The model under review builds one solid part; all positions refer to its coordinate system, in mm. Face numbers are marked on the shaded views. A direction names the side the tool comes from. Coordinates: 2 decimals unless noted, no trailing zeros. Order: outer loops, then holes, each group sorted by start corner. A loop starts at its lowest first (then second) coordinate and runs counter-clockwise, first axis right, second up. Notation, with made-up numbers: (46, 9.5) - (57, 9.5) arc R29 ccw to (57, 42.5) - close; hole circle Ø1 at (-9.75, 41). An arc over 180 degrees is marked (long way). Answer in a Markdown table with one row per item.
```python
from build123d import *

# Parameters (mm, degrees)
BOSS_EXTRUDE1_DEPTH          = 44.45
FILLET2_R                    = 6.35
CUT_EXTRUDE1_START           = -22.225
CUT_EXTRUDE1_DEPTH           = 22.225
FILLET3_R                    = 2.54
F_3_8_0_375_DIAMETER_HOLE1_D = 10.16


with BuildPart() as part:
    # Sketch1 → Boss-Extrude1 (new body)
    with BuildSketch(Plane.XY):
        with BuildLine():
            Line((0, 0), (57.15, 0))
            Line((57.15, 0), (57.15, -9.525))
            Line((57.15, -9.525), (0, -11.7445024))
            Line((0, -11.7445024), (-20.4502, -11.7445024))
            Line((-20.4502, -11.7445024), (-20.4502, 9.8454976))
            Line((-20.4502, 9.8454976), (-48.3902, 9.8454976))
            Line((-48.3902, 9.8454976), (-48.3902, 20.0054976))
            ThreePointArc((-48.3902, 20.0054976), (-44.670456121, 28.985753721), (-35.6902, 32.7054976))
            Line((-35.6902, 32.7054976), (-22.9902, 32.7054976))
            Line((-22.9902, 32.7054976), (-6.35, 57.15))
            Line((-6.35, 57.15), (0, 57.15))
            Line((0, 57.15), (0, 0))
        make_face()
    extrude(amount=BOSS_EXTRUDE1_DEPTH)

    # Fillet2
    fillet2_edges = [part.edges().sort_by_distance(p)[0] for p in [
        (0, 0, 22.225),
    ]]
    fillet(fillet2_edges, radius=FILLET2_R)

    # Sketch3 → Cut-Extrude1 (cut)
    with BuildSketch(Plane.XY.offset(44.45).offset(CUT_EXTRUDE1_START)):
        with BuildLine():
            Line((-48.3902, 9.8454976), (-20.4502, 9.8454976))
            Line((-20.4502, 9.8454976), (-20.4502, 36.436765018))
            Line((-20.4502, 36.436765018), (-22.9902, 32.7054976))
            Line((-22.9902, 32.7054976), (-35.6902, 32.7054976))
            ThreePointArc((-35.6902, 32.7054976), (-44.670456121, 28.985753721), (-48.3902, 20.0054976))
            Line((-48.3902, 20.0054976), (-48.3902, 9.8454976))
        make_face()
    extrude(amount=CUT_EXTRUDE1_DEPTH, mode=Mode.SUBTRACT)

    # Fillet3
    fillet3_edges = [part.edges().sort_by_distance(p)[0] for p in [
        (-22.9902, 32.7054976, 11.1125),
    ]]
    fillet(fillet3_edges, radius=FILLET3_R)

    # 3/8 (0.375) Diameter Hole1 (through all)
    with Locations(Plane(origin=(0, 0, 0), x_dir=(-1, 0, 0), z_dir=(0, 0, -1))):
        with Locations((35.6902, 21.2754976)):
            Hole(F_3_8_0_375_DIAMETER_HOLE1_D / 2)


solid = part.part
```
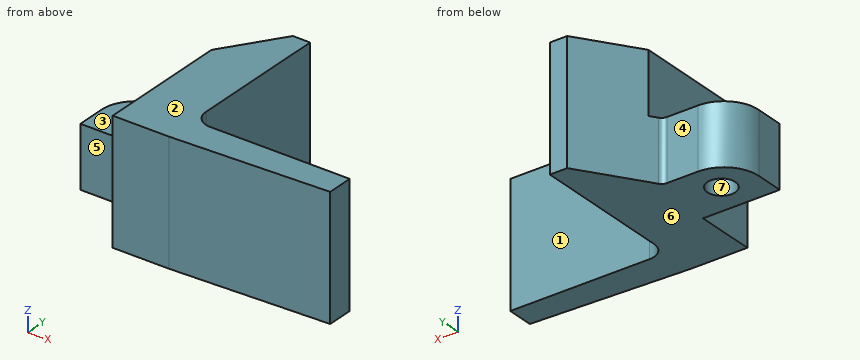
Item 1: Mouldability with a two-part tool opening along Y and no side actions: class the marked faces 4, 5, 6 and 7 as +Y half, -Y half, draft (parallel to the pull), parting line (faces both ways), or undercut.
Check values:
| item | result |
|---|---|
| face 4 | +Y half |
| face 5 | -Y half |
| face 6 | draft |
| face 7 | undercut |
Item 2: We need section A-A, the plane x = -38. Write out the cut boundary in (y, z) (1 decimal).
Check values:
| item | result |
|---|---|
| outline | (9.8, 0) - (16.8, 0) - (16.8, 22.2) - (9.8, 22.2) - close; (25.8, 0) - (32.5, 0) - (32.5, 22.2) - (25.8, 22.2) - close |
Item 3: Clearance check with flat-ended pins moving along their axes: pin 1 Ø12.5 at (x, z) = (-27.5, 16.5) entering from +Y; pin 2 Ø1 at (x, y) = (-17, 39.5) entering from -Z; pin 3 Ø4 at (y, z) = (35, 7.5) entering from -X; pin 4 Ø2 at (x, z) = (35.5, 31.5) entering from -Y. State where each tip first meets the part, or that it passes through.
Check values:
| item | result |
|---|---|
| pin 1 | y = 35.26 |
| pin 2 | z = 0 |
| pin 3 | x = -23.15 |
| pin 4 | y = -10.4 |
Item 4: To check wall thickness, follow line 1 (X direction, y = -6.5, z = 16); line 2 (X direction, y = 23, z = 38.5); line 3 (Y direction, x = 14, z = 11.5). State the ranges of each line that lie inside material, in increasing order. Write a range as from..to.
Check values:
| item | result |
|---|---|
| line 1 | -20.45..57.15 |
| line 2 | -20.45..0 |
| line 3 | -11.2..0 |
Item 5: We need section C-C, the plane y = -1.5. Write out the cut boundary in (x, z).
Check values:
| item | result |
|---|---|
| outline | (-20.45, 0) - (57.15, 0) - (57.15, 44.45) - (-20.45, 44.45) - close |
Item 6: Tool access review of the marked faces 1, 2 and 3: name each direction out of +Z, -Z, +X, -X, +Y, -Y from which nothing blocks a thin tool from reaching the whole face with its end or side.
Check values:
| item | result |
|---|---|
| face 1 | +Z, -Z, +X, +Y |
| face 2 | +Z, +X, -X, +Y, -Y |
| face 3 | +Z, -X, +Y, -Y |
